Geometry check sheet. Reference: the model listing, model coordinates, mm. Give positions to 0.01 mm unless a question says otherwise; leave off trailing zeros. Write each loop counter-clockwise with the first axis right and the second up, starting at its lowest first coordinate (ties: lowest second). Pieces come first, ordered by that corner, then holes. Notation, with made-up numbers: (47, 57) -> (101, 57) arc R25 cw to (101, 72) -> close; hole circle Ø5 at (41.5, -8). An arc over 180 degrees is marked (long way). Write item = value, one per line. Start each with the question number.
1. Thickness scan on line 1 along Z through (x, y) = (-111, 1.1); line 2 along Z through (x, y) = (107.5, 0.4); line 3 along X through (y, z) = (-0.55, -116.5). Record the ranges inside material, lowest first.
2. Cross-section at A-A, the plane x = -71.5. Record the cut outline in (y, z).
3. Depth check by flat-ended pin: P1, Ø0.9, axis at y = -0.5, z = -127.5, coming from the +X side; P2, Ø1.5, axis at x = 0, y = 0, coming from the -Z side. Enter the tip coordinate at first touch or a pass-through.
4. Cross-section at B-B, the plane z = -9.5. Record the cut outline in (x, y).
```python
from build123d import *

# Parameters (mm, degrees)
SALIENTE_EXTRUIR1_DEPTH = 1.5
CORTAR_EXTRUIR1_DEPTH   = 3
MATRIZC1_COUNT          = 3
CORTAR_EXTRUIR4_REACH   = 5


with BuildPart() as part:
    # Croquis1 → Saliente-Extruir1 (new body, symmetric)
    with BuildSketch(Plane(origin=(0, 0, 0), x_dir=(1, 0, 0), z_dir=(0, 1, 0))):
        with BuildLine():
            Line((-129.903810568, -55), (-17.320508076, 140))
            ThreePointArc((-17.320508076, 140), (0, 150), (17.320508076, 140))
            Line((17.320508076, 140), (129.903810568, -55))
            ThreePointArc((129.903810568, -55), (129.903810568, -75), (112.583302492, -85))
            Line((112.583302492, -85), (-112.583302492, -85))
            ThreePointArc((-112.583302492, -85), (-129.903810568, -75), (-129.903810568, -55))
        make_face()
    extrude(amount=SALIENTE_EXTRUIR1_DEPTH, both=True)

    # Croquis2 → Cortar-Extruir1 (cut)
    with BuildSketch(Plane(origin=(0, 1.5, 0), x_dir=(1, 0, 0), z_dir=(0, 1, 0))):
        Polygon((107.503175473, -63.799038106), (109.003175473, -61.200961894), (100.342921435, -56.200961894), (98.842921435, -58.799038106), align=None)
        Polygon((113.784264386, -59.919872981), (116.382340598, -61.419872981), (121.382340598, -52.759618943), (118.784264386, -51.259618943), align=None)
        Polygon((117.663429511, -66.200961894), (116.163429511, -68.799038106), (124.823683549, -73.799038106), (126.323683549, -71.200961894), align=None)
        Polygon((111.382340598, -70.080127019), (108.784264386, -68.580127019), (103.784264386, -77.240381057), (106.382340598, -78.740381057), align=None)
    cortar_extruir1 = extrude(amount=-CORTAR_EXTRUIR1_DEPTH, mode=Mode.SUBTRACT)

    # MatrizC1: Cortar-Extruir1 ×3 about axis
    matrizc1_axis = Axis((-0.369121776, 0, -0.213112557), (0, 1, 0))
    for i in range(1, MATRIZC1_COUNT):
        add(cortar_extruir1.rotate(matrizc1_axis, i * 360 / MATRIZC1_COUNT), mode=Mode.SUBTRACT)

    # Croquis5 → Cortar-Extruir4 (cut, up to next)
    with BuildSketch(Plane(origin=(0, 1.5, 0), x_dir=(1, 0, 0), z_dir=(0, 1, 0)), mode=Mode.PRIVATE) as cortar_extruir4_sk1:
        Polygon((-123.633404248, -44.139337671), (-112.772507939, -62.950961894), (-109.741419026, -61.200961894), (-108.241419026, -63.799038106), (-111.272507939, -65.549038106), (-100.042489853, -85), (-147.224318643, -85), align=None)
    cortar_extruir4_tool1 = extrude(cortar_extruir4_sk1.sketch, amount=-CORTAR_EXTRUIR4_REACH, mode=Mode.PRIVATE) & part.part
    add(cortar_extruir4_tool1.solids().sort_by_distance((-123.491961, 1.5, 71.293524))[0], mode=Mode.SUBTRACT)
    # Croquis5 → Cortar-Extruir4 (cut, up to next)
    with BuildSketch(Plane(origin=(0, 1.5, 0), x_dir=(1, 0, 0), z_dir=(0, 1, 0)), mode=Mode.PRIVATE) as cortar_extruir4_sk2:
        Polygon((-1.869121776, 129.139337671), (-23.590914395, 129.139337671), (0, 170), (23.590914395, 129.139337671), (1.130878224, 129.139337671), (1.130878224, 125.639337671), (-1.869121776, 125.639337671), align=None)
    cortar_extruir4_tool2 = extrude(cortar_extruir4_sk2.sketch, amount=-CORTAR_EXTRUIR4_REACH, mode=Mode.PRIVATE) & part.part
    add(cortar_extruir4_tool2.solids().sort_by_distance((-0.003977, 1.5, -142.593938))[0], mode=Mode.SUBTRACT)
    # Croquis5 → Cortar-Extruir4 (cut, up to next)
    with BuildSketch(Plane(origin=(0, 1.5, 0), x_dir=(1, 0, 0), z_dir=(0, 1, 0)), mode=Mode.PRIVATE) as cortar_extruir4_sk3:
        Polygon((112.034264386, -62.950961894), (123.264282472, -43.5), (147.224318643, -85), (99.304246301, -85), (110.534264386, -65.549038106), (107.503175473, -63.799038106), (109.003175473, -61.200961894), align=None)
    cortar_extruir4_tool3 = extrude(cortar_extruir4_sk3.sketch, amount=-CORTAR_EXTRUIR4_REACH, mode=Mode.PRIVATE) & part.part
    add(cortar_extruir4_tool3.solids().sort_by_distance((123.123262, 1.5, 71.085248))[0], mode=Mode.SUBTRACT)


solid = part.part
```
Answers:
q1.line_1 = 22.26 to 61.93, 65.39 to 66.02
q1.line_2 = 16.2 to 60.33, 63.8 to 70.8
q1.line_3 = -30.89 to -1.87, 1.13 to 30.89
q2.outline = (-1.5, -46.16) -> (1.5, -46.16) -> (1.5, 85) -> (-1.5, 85) -> close
q3.P1 = 24.8
q3.P2 = -115.64
q4.outline = (-92.66, -1.5) -> (92.66, -1.5) -> (92.66, 1.5) -> (-92.66, 1.5) -> close
